Work out the finished part from the listing and answer in its coordinate system (mm). A direction names the side the tool comes from. Give positions to 0.01 mm unless a question says otherwise; leave off trailing zeros. Loops run counter-clockwise (first coordinate to the right, second up) from the corner with the lowest first, then second, coordinate; pieces in that order, holes last. Notation, with made-up numbers: M -29,49.5 L 11,49.5 A14 ccw 11,64.5 Z; hole C 37.5,5 d8. An arc over 180 degrees is marked long. Answer as a JSON object with one key per item and string values. Group by question number.
```python
from build123d import *

# Parameters (mm, degrees)
F1_DEPTH    = 35
F2_R        = 7.5
F3_DEPTH    = 5
F4_R        = 1
F5_W        = 20
F5_H        = 20
F6_DEPTH    = 35.001
F7_T        = 7.5
F7_T3_DEPTH = 50
F10_DEPTH   = 10
F9_R        = 6
F11_DEPTH   = 200


# Not quite as in the source:
# - a shell that OpenCascade refuses in one call is made with other operations: the cavity is built on its own and cut out


with BuildPart() as f1:
    # F0 (on Top) → F1 (new body)
    with BuildSketch(Plane.XY):
        Polygon((25, 43.3012701892), (-25, 43.3012701892), (-50, 0), (-25, -43.3012701892), (25, -43.3012701892), (50, 0), align=None)
    extrude(amount=F1_DEPTH)

    # F2 (on face) → F3 (join)
    with BuildSketch(Plane.XY.offset(35)):
        with Locations((0, 21.6506350946)):
            Circle(F2_R)
    extrude(amount=F3_DEPTH)

    # F4
    f4_edges = [f1.edges().sort_by_distance(p)[0] for p in [
        (-7.5, 21.650635, 40),
    ]]
    fillet(f4_edges, radius=F4_R)

    # F5 (on face) → F6 (cut, through all)
    with BuildSketch(Plane.XY.offset(35)):
        with Locations((-50, 0)):
            Rectangle(F5_W, F5_H)
    extrude(amount=-F6_DEPTH, mode=Mode.SUBTRACT)

    # F7: shell of thickness 7.5, made by hand


with BuildPart() as f7_core1:
    # F7_t2: copy of F1
    add(f1.part)

    # the walls: a layer under each face that stays
    f7_faces = [f7_core1.faces().sort_by_distance(p)[0] for p in [
        (2.8867513459, 0, 35),
        (0, 21.6506350946, 40),
        (37.5, 21.6506350946, 17.5),
        (37.5, -21.6506350946, 17.5),
        (0, -43.3012701892, 17.5),
        (-34.6132486541, -26.6506350946, 17.5),
        (-42.1132486541, -10, 17.5),
        (-40, 0, 17.5),
        (-42.1132486541, 10, 17.5),
        (-34.6132486541, 26.6506350946, 17.5),
        (0, 43.3012701892, 17.5),
    ]]
    thicken(f7_faces, amount=-F7_T, mode=Mode.SUBTRACT)

    # F7_s4 → F7_t3 (cut)
    with BuildSketch(Plane.XY.offset(-7.5)):
        Polygon((-40.075, -9.925), (-40, -17.5), (-32.5, -17.5), (-32.5, -10), align=None)
        Polygon((-40.075, 9.925), (-32.5, 10), (-32.5, 17.5), (-40, 17.5), align=None)
    extrude(amount=F7_T3_DEPTH, mode=Mode.SUBTRACT)

    # F7_s5 → F7_t6 (revolve, cut)
    with BuildSketch(Plane.XZ.offset(-21.6506350946)):
        Polygon((7.575, 35.075), (0, 35), (0, 27.5), (7.5, 27.5), align=None)
    revolve(axis=Axis((0, 21.6506350946, 35), (0, 0, 1)), mode=Mode.SUBTRACT)


with BuildPart() as f1_1:
    add(f1.part)

    # what is left inside the walls is the cavity
    f7_cavity = [f7_core1.part.solids().sort_by_distance(p)[0] for p in [
        (4.419873, -11.933757, 27.425),
    ]]
    add(f7_cavity, mode=Mode.SUBTRACT)

    # F8 (on Front) → F10 (join, symmetric)
    with BuildSketch(Plane.XZ):
        Polygon((-10, 6.8261531631), (-10, 26.8261531631), (-70, 26.8261531631), (-90, 17.5), (-79.3261531631, 6.8261531631), (-54.9282032303, 6.8261531631), (-49.7320508076, 3.8261531631), (-48, 6.8261531631), align=None)
    extrude(amount=F10_DEPTH, both=True)

    # F9 (on Right) → F11 (join)
    with BuildSketch(Plane.YZ):
        with Locations((0, 17.5)):
            Circle(F9_R)
    extrude(amount=-F11_DEPTH)


solid = f1_1.part
```
Item 1: A cutting plane is placed at C-C (x = -73.5). Determine the outline of the cut face in (y, z).
Item 2: Find the intervals of material crossed by probe 1 along Y at (x, z) = (-17, 15.5); probe 2 along Z at (x, y) = (-18.5, 7); probe 3 along Y at (x, z) = (-28.5, 21.5), in increasing order. Write a range as [from, to].
Item 3: Given pin 1 Ø7 at (x, z) = (-60, 13.5) entering from +Y; pin 2 Ø5 at (y, z) = (-16.5, 21) entering from +X; pin 3 Ø4.5 at (x, z) = (-42, 33) entering from -Y, each flat-ended and moving along its own axis, determine where each tip first touches the part or whether it passes through.
Item 4: A tool of negligible diameter and unlimited length cuts with its end or side. For faces 4 (the flat face through (30.86, -18.15, 13.56)), 5 (the flat face through (-10, 4, 12)), 6 (the flat face through (-42, 10, 31)), 7 (the flat face through (-62, -10, 15)), 8 (the flat face through (37.675, 21.348, 17.255)), from which of +Z, -Z, +X, -X, +Y, -Y can it reach the whole face along a straight path? Write none if from no direction.
Item 5: A cutting plane is placed at A-A (z = 14.5). Determine the outline of the cut face in (x, y).
Item 6: A cutting plane is placed at B-B (x = -166.5). Determine the outline of the cut face in (y, z), and give its area (3 significant figures).
Item 7: For a pull along Y with two mould halves and no side action, classify faces 1 (the cylindrical face through (-1.63, 14.33, 36.97)), 2 (the flat face through (-44, 0, 6.826)), 3 (the flat face through (2, 1, 35)) as pulls with the +Y half, pulls with the -Y half, needs draft (parallel to the pull), parting line crosses it, or undercut.
The answers:
{
 "1": {"outline": "M -10,6.83 L 10,6.83 L 10,25.19 L -10,25.19 Z"},
 "2": {"probe 1": "y = [-43.3, -35.8], [-10, 10], [35.8, 43.3]", "probe 2": "z = [6.83, 26.83], [27.5, 35]", "probe 3": "y = [-37.24, -22.24], [-10, 10], [22.24, 37.24]"},
 "3": {"pin 1": "stops at y = 10", "pin 2": "stops at x = 41.92", "pin 3": "stops at y = -17.75"},
 "4": {"face 4": "-Z", "face 5": "none", "face 6": "+Z, -X", "face 7": "+Z, -Z, -X, -Y", "face 8": "+Z, -Z, +X, +Y"},
 "5": {"outline": "M -200,-5.2 L -87,-5.2 L -87,-10 L -44.23,-10 L -25,-43.3 L 25,-43.3 L 50,0 L 25,43.3 L -25,43.3 L -44.23,10 L -87,10 L -87,5.2 L -200,5.2 Z; hole M -32.5,-15.31 L -20.67,-35.8 L 20.67,-35.8 L 41.34,0 L 20.67,35.8 L -20.67,35.8 L -32.5,15.31 L -32.5,10 L -10,10 L -10,5.2 L 0,5.2 L 0,-5.2 L -10,-5.2 L -10,-10 L -32.5,-10 Z"},
 "6": {"outline": "C 0,17.5 d12", "area": "113 mm^2"},
 "7": {"face 1": "parting line crosses it", "face 2": "undercut", "face 3": "needs draft"}
}
